The model under review builds one solid part; all positions refer to its coordinate system, in mm. A direction names the side the tool comes from. Coordinates: 2 decimals unless noted, no trailing zeros. Order: outer loops, then holes, each group sorted by start corner. A loop starts at its lowest first (then second) coordinate and runs counter-clockwise, first axis right, second up. Notation, with made-up numbers: M -26,-22.75 L 31,-22.75 A16 ccw 31,-17.75 Z; hole C -38.5,45 d6. An arc over 180 degrees is marked long. Answer as CSV lines item,"result". Start each with the question number.
Q1. For P1, Ø2.5, axis at x = 1.5, z = -9, coming from the -Y side; P2, Ø1.5, axis at x = -2.5, y = 5.5, coming from the -Z side; P3, Ø2.5, axis at x = -0.5, y = 9, coming from the +Z side, all flat-tipped, find the tip position at first contact; note any pin that passes through.
Q2. Consider section A-A on z = 0. Write out the cut boundary in (x, y).
Q3. Consider section C-C on y = 0.5. Write out the cut boundary in (x, z).
Q4. Wall thickness on L1, parallel to Y at x = 0.5, z = 0; L2, parallel to X at y = 14.85, z = 10; L3, parallel to Y at x = 1.25, z = 11.5: over which ranges is each line inside the solid? List them lowest first. Write a range as [from, to].
Q5. Machinability: for faces 1 (the face through (0, 17, 0)), 2 (the face through (2, 12, -10)), 3 (the face through (2, 12, 10)), which of the approach directions +Z, -Z, +X, -X, +Y, -Y give a long, thin tool a straight path to every point of the face, cutting with its end or side? Answer none if there is none.
Q6. The part is to be moulded in two halves that separate along Z. For faces 4 (the face through (0, 15, 15)), 5 (the face through (-4, 9, 0)), 6 (the face through (-0.06, 0.07, 1.5)), 7 (the face through (0, 6, -5)), say which applies: +Z half, -Z half, draft (parallel to the pull), parting line (faces both ways), or undercut.
Q7. Consider section D-D on y = 12.5. Write out the cut boundary in (x, z).
Q8. Consider section B-B on x = 2. Write out the cut boundary in (y, z), and give its area (3 significant figures).
from build123d import *

# Parameters (mm, degrees)
SKETCH_1_R          = 1.5
EXTRUDE_1_DEPTH     = 4
CUT_EXTRUDE_1_REACH = 25.022
SKETCH_2_R          = 1.5


with BuildPart() as part:
    # 草图1 → 凸台-拉伸1 (new, symmetric)
    with BuildSketch(Plane(origin=(0, 0, 0), x_dir=(0, 0, -1), z_dir=(1, 0, 0))):
        with BuildLine():
            Line((5, 12), (15, 12))
            Line((15, 12), (15, 17))
            Line((15, 17), (-15, 17))
            Line((-15, 17), (-15, 12))
            Line((-15, 12), (-5, 12))
            Line((-5, 12), (-5, 0))
            ThreePointArc((-5, 0), (0, -5), (5, 0))
            Line((5, 0), (5, 12))
        make_face()
        Circle(SKETCH_1_R, mode=Mode.SUBTRACT)
    extrude(amount=EXTRUDE_1_DEPTH, both=True)

    # 草图2 → 切除-拉伸1 (cut, up to next)
    with BuildSketch(Plane.XZ.offset(-12), mode=Mode.PRIVATE) as cut_extrude_1_sk1:
        with Locations(Location((0, 10, 0), (0, 0, 270))):
            Circle(SKETCH_2_R)
    cut_extrude_1_tool1 = extrude(cut_extrude_1_sk1.sketch, amount=-CUT_EXTRUDE_1_REACH, mode=Mode.PRIVATE) & part.part
    # 草图2 → 切除-拉伸1 (cut, up to next)
    with BuildSketch(Plane.XZ.offset(-12), mode=Mode.PRIVATE) as cut_extrude_1_sk2:
        with Locations(Location((0, -10, 0), (0, 0, 270))):
            Circle(SKETCH_2_R)
    cut_extrude_1_tool2 = extrude(cut_extrude_1_sk2.sketch, amount=-CUT_EXTRUDE_1_REACH, mode=Mode.PRIVATE) & part.part
    add(cut_extrude_1_tool1.solids().sort_by_distance((0, 12, 10))[0], mode=Mode.SUBTRACT)
    add(cut_extrude_1_tool2.solids().sort_by_distance((0, 12, -10))[0], mode=Mode.SUBTRACT)


solid = part.part
Evaluation:
1,P1,"stops at y = 12"
1,P2,"stops at z = -5"
1,P3,"stops at z = 5"
2,outline,"M -4,-5 L 4,-5 L 4,-1.5 L -4,-1.5 Z; M -4,1.5 L 4,1.5 L 4,17 L -4,17 Z"
3,outline,"M -4,-5 L 4,-5 L 4,-1.41 L -4,-1.41 Z; M -4,1.41 L 4,1.41 L 4,5 L -4,5 Z"
4,L1,"y = [-5, -1.5], [1.5, 17]"
4,L2,"x = [-4, -1.5], [1.5, 4]"
4,L3,"y = [12, 17]"
5,face 1,"+Z, -Z, +X, -X, +Y"
5,face 2,"-Z, +X, -X, -Y"
5,face 3,"+Z, +X, -X, -Y"
6,face 4,"+Z half"
6,face 5,"draft"
6,face 6,"undercut"
6,face 7,"-Z half"
7,outline,"M -4,-15 L 4,-15 L 4,15 L -4,15 Z; hole C 0,-10 d3; hole C 0,10 d3"
8,outline,"M 0,-5 L 12,-5 L 12,-15 L 17,-15 L 17,15 L 12,15 L 12,5 L 0,5 A5 ccw Z; hole C 0,0 d3"
8,area,"302 mm²"
